```python
from build123d import *

# Parameters (mm, degrees)
F1_DEPTH = 3
F2_DEPTH = 9
F3_DEPTH = 9.001


with BuildPart() as f1:
    # F0 (on Top) → F1 (new body)
    with BuildSketch(Plane.XY):
        with BuildLine():
            Line((-5.4486236794, 0.75), (-8.4668471109, 0.75))
            ThreePointArc((-8.4668471109, 0.75), (-8.4917077329, 0.3753661926), (-8.5, 0))
            Line((-8.5, 0), (-5.5, 0))
            ThreePointArc((-5.5, 0), (-5.4871408874, 0.3758788124), (-5.4486236794, 0.75))
        make_face()
        with BuildLine():
            ThreePointArc((-8.5, 0), (0, -8.5), (8.5, 0))
            ThreePointArc((8.5, 0), (0.3753661926, 8.4917077329), (-8.4668471109, 0.75))
            Line((-8.4668471109, 0.75), (-5.4486236794, 0.75))
            ThreePointArc((-5.4486236794, 0.75), (0.3758788124, 5.4871408874), (5.5, 0))
            ThreePointArc((5.5, 0), (0, -5.5), (-5.5, 0))
            Line((-5.5, 0), (-8.5, 0))
        make_face()
        with BuildLine():
            ThreePointArc((-8.5, 0), (-8.4917077329, 0.3753661926), (-8.4668471109, 0.75))
            Line((-8.4668471109, 0.75), (-11.4755174175, 0.75))
            ThreePointArc((-11.4755174175, 0.75), (-11.4938777247, 0.3751997458), (-11.5, 0))
            Line((-11.5, 0), (-8.5, 0))
        make_face()
        with BuildLine():
            ThreePointArc((-8.4668471109, 0.75), (0.3753661926, 8.4917077329), (8.5, 0))
            ThreePointArc((8.5, 0), (0, -8.5), (-8.5, 0))
            Line((-8.5, 0), (-11.5, 0))
            ThreePointArc((-11.5, 0), (0, -11.5), (11.5, 0))
            ThreePointArc((11.5, 0), (0.3751997458, 11.4938777247), (-11.4755174175, 0.75))
            Line((-11.4755174175, 0.75), (-8.4668471109, 0.75))
        make_face()
    extrude(amount=F1_DEPTH)

    # F0 (on Top) → F2 (join)
    with BuildSketch(Plane.XY):
        with BuildLine():
            ThreePointArc((-8.5, 0), (-8.4917077329, 0.3753661926), (-8.4668471109, 0.75))
            Line((-8.4668471109, 0.75), (-11.4755174175, 0.75))
            ThreePointArc((-11.4755174175, 0.75), (-11.4938777247, 0.3751997458), (-11.5, 0))
            Line((-11.5, 0), (-8.5, 0))
        make_face()
        with BuildLine():
            ThreePointArc((-8.4668471109, 0.75), (0.3753661926, 8.4917077329), (8.5, 0))
            ThreePointArc((8.5, 0), (0, -8.5), (-8.5, 0))
            Line((-8.5, 0), (-11.5, 0))
            ThreePointArc((-11.5, 0), (0, -11.5), (11.5, 0))
            ThreePointArc((11.5, 0), (0.3751997458, 11.4938777247), (-11.4755174175, 0.75))
            Line((-11.4755174175, 0.75), (-8.4668471109, 0.75))
        make_face()
    extrude(amount=F2_DEPTH)

    # F0 (on Top) → F3 (cut, through all)
    with BuildSketch(Plane.XY):
        with BuildLine():
            Line((-5.4486236794, 0.75), (-8.4668471109, 0.75))
            ThreePointArc((-8.4668471109, 0.75), (-8.4917077329, 0.3753661926), (-8.5, 0))
            Line((-8.5, 0), (-5.5, 0))
            ThreePointArc((-5.5, 0), (-5.4871408874, 0.3758788124), (-5.4486236794, 0.75))
        make_face()
        with BuildLine():
            ThreePointArc((-8.5, 0), (-8.4917077329, 0.3753661926), (-8.4668471109, 0.75))
            Line((-8.4668471109, 0.75), (-11.4755174175, 0.75))
            ThreePointArc((-11.4755174175, 0.75), (-11.4938777247, 0.3751997458), (-11.5, 0))
            Line((-11.5, 0), (-8.5, 0))
        make_face()
    extrude(amount=F3_DEPTH, mode=Mode.SUBTRACT)


solid = f1.part
```
Model file for the job. Use its own axes, mm. A direction names the side the tool comes from. Round coordinates to 2 decimals unless told otherwise and drop trailing zeros. Loops run counter-clockwise (first coordinate to the right, second up) from the corner with the lowest first, then second, coordinate; pieces in that order, holes last. Notation, with made-up numbers: M -19,4 L 1,4 A13 ccw 1,11 Z; hole C 67.5,-20.5 d1. An arc over 180 degrees is marked long. Put each result on its own line as item: value. Start each with the question number.
Item 1: Cut at C-C (z = 4.5). List the corners of the cut face in (x, y), then the cut area to 3 significant figures.
Item 2: 3-axis set-ups, long thin cutter, end or side, ignore diameter. For faces 4 (the face through (-9, 0, 3)), 5 (the face through (5, 3, 0)): which of +Z, -Z, +X, -X, +Y, -Y reach the whole face in a straight line?
Item 3: Cut at D-D (x = 8). List the corners of the cut face in (y, z).
Item 4: Cut at A-A (x = 0). List the corners of the cut face in (y, z), then the cut area to 3 significant figures.
Item 5: Cut at B-B (y = -2.5). List the corners of the cut face in (x, z).
Item 6: Drop flat-ended pins along their axis: P1, Ø1.8, axis at x = -9, z = 4, coming from the +Y side; P2, Ø3, axis at x = -9.5, z = 5, coming from the -Y side. Give the stop position or say it passes through.
Item 7: Mould opens along X. For faces 1 (the face through (11.467, -0.875, 4.437)), 2 (the face through (6, 0, 3)), 3 (the face through (-9, 0.75, 3)) say: released by +X, released by -X, zero draft, split by the parting line, or undercut.
Item 8: Drill centre lines: line 1 along X through (y, z) = (2, 7.75); line 2 along Y through (x, z) = (4.5, 2); line 3 along Z through (x, y) = (6.75, 0.25). Where is each one in solid material? Low to high.
Answer block:
1. outline: M -11.5,0 A11.5 ccw long -11.48,0.75 L -8.47,0.75 A8.5 cw long -8.5,0 Z
1. area: 186 mm2
2. face 4: +Z, -Z, -X
2. face 5: -Z, +X, -X, +Y, -Y
3. outline: M -8.26,0 L 8.26,0 L 8.26,9 L 2.87,9 L 2.87,3 L -2.87,3 L -2.87,9 L -8.26,9 Z
4. outline: M -11.5,0 L -5.5,0 L -5.5,3 L -8.5,3 L -8.5,9 L -11.5,9 Z; M 5.5,0 L 11.5,0 L 11.5,9 L 8.5,9 L 8.5,3 L 5.5,3 Z
4. area: 72.0 mm2
5. outline: M -11.22,0 L -4.9,0 L -4.9,3 L -8.12,3 L -8.12,9 L -11.22,9 Z; M 4.9,0 L 11.22,0 L 11.22,9 L 8.12,9 L 8.12,3 L 4.9,3 Z
6. P1: y = 8.16
6. P2: y = -8.26
7. face 1: split by the parting line
7. face 2: undercut
7. face 3: zero draft
8. line 1: -11.32 to -8.26, 8.26 to 11.32
8. line 2: -10.58 to -3.16, 3.16 to 10.58
8. line 3: 0 to 3
